The model under review builds one solid part; all positions refer to its coordinate system, in mm. Give positions to 0.01 mm unless a question says otherwise; leave off trailing zeros. Order: outer loops, then holes, each group sorted by start corner. A loop starts at its lowest first (then second) coordinate and runs counter-clockwise, first axis right, second up. Notation, with made-up numbers: (77, -2.75) - (117, -2.75) arc R24 ccw to (117, 28.25) - close; hole circle Ø3 at (-26, 31). An arc over 180 degrees is marked (long way). Use a Markdown table: item, result. Add a question column.
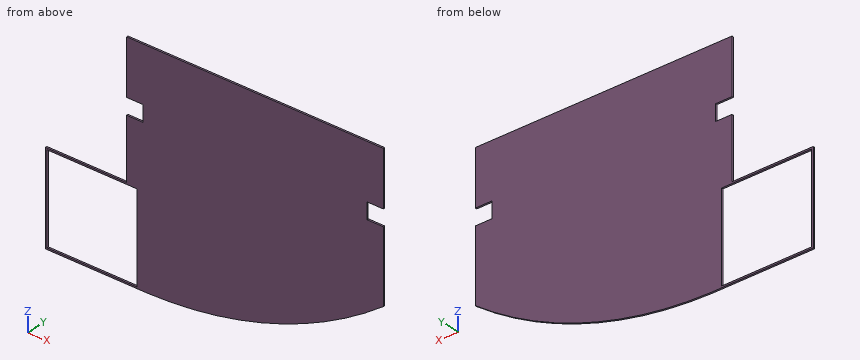
```python
from build123d import *

# Parameters (mm, degrees)
F0_W     = 139.7
F0_H     = 139.7
F1_DEPTH = 2.54
F2_W     = 25.4
F2_H     = 25.4
F3_DEPTH = 25.4
F4_W     = 25.4
F4_H     = 25.4
F5_DEPTH = 25.4


with BuildPart() as f1:
    # F0 (on Front) → F1 (new body)
    with BuildSketch(Plane.XZ):
        with BuildLine():
            Line((300.720289, 79.205069), (-98.059711, 79.205069))
            Line((-98.059711, 79.205069), (-98.059711, -128.566931))
            Line((-98.059711, -128.566931), (-224.297711, -128.566931))
            Line((-224.297711, -128.566931), (-224.297711, -273.346931))
            Line((-224.297711, -273.346931), (-82.057711, -273.346931))
            Line((-82.057711, -273.346931), (-64.778368, -273.346931))
            ThreePointArc((-64.778368, -273.346931), (128.230167, -239.372335), (300.720289, -146.346931))
            Line((300.720289, -146.346931), (300.720289, 79.205069))
        make_face()
        with Locations((-151.907711, -200.956931)):
            Rectangle(F0_W, F0_H, mode=Mode.SUBTRACT)
    extrude(amount=F1_DEPTH)

    # F2 (on face) → F3 (cut)
    with BuildSketch(Plane.XZ.offset(2.54)):
        with Locations((-85.359711, -19.854931)):
            Rectangle(F2_W, F2_H)
    extrude(amount=-F3_DEPTH, mode=Mode.SUBTRACT)

    # F4 (on face) → F5 (cut)
    with BuildSketch(Plane.XZ.offset(2.54)):
        with Locations((288.020289, -19.854931)):
            Rectangle(F4_W, F4_H)
    extrude(amount=-F5_DEPTH, mode=Mode.SUBTRACT)


solid = f1.part
```
Q1. Wall thickness on probe 1 along Z at (x, y) = (-137, -0.3); probe 2 along X at (y, z) = (-1.8, -197); probe 3 along X at (y, z) = (-1, -211.5): over which ranges is each line inside the solid? List them lowest first.
Q2. We need section C-C (x = 14.5). Write out the cut boundary in (y, z), plus the area to 3 significant figures.
Q3. Clearance check with flat-ended pins moving along their axes: P1, Ø0.8, axis at y = -1, z = -22.5, coming from the -X side; P2, Ø0.8, axis at x = -165, y = -0.5, coming from the +Z side; P3, Ø1.3, axis at y = -1.5, z = -101, coming from the -X side. State where each tip first meets the part, or that it passes through.
Q4. We need section B-B (y = -1.6). Write out the cut boundary in (x, z).
Q5. We need section D-D (x = 112.5). Write out the cut boundary in (y, z), plus the area to 3 significant figures.
Q6. We need section A-A (x = -106.5). Write out the cut boundary in (y, z), plus the area to 3 significant figures.
Here are the results:
| question | item | result |
|---|---|---|
| 1 | probe 1 | -273.35 to -270.81, -131.11 to -128.57 |
| 1 | probe 2 | -224.3 to -221.76, -82.06 to 223.31 |
| 1 | probe 3 | -224.3 to -221.76, -82.06 to 195.35 |
| 2 | outline | (-2.54, -267.08) - (0, -267.08) - (0, 79.21) - (-2.54, 79.21) - close |
| 2 | area | 880 mm2 |
| 3 | P1 | x = -72.66 |
| 3 | P2 | z = -128.57 |
| 3 | P3 | x = -98.06 |
| 4 | outline | (-224.3, -273.35) - (-64.78, -273.35) arc R614.37 ccw to (300.72, -146.35) - (300.72, -32.55) - (275.32, -32.55) - (275.32, -7.15) - (300.72, -7.15) - (300.72, 79.21) - (-98.06, 79.21) - (-98.06, -7.15) - (-72.66, -7.15) - (-72.66, -32.55) - (-98.06, -32.55) - (-98.06, -128.57) - (-224.3, -128.57) - close; hole (-221.76, -270.81) - (-82.06, -270.81) - (-82.06, -131.11) - (-221.76, -131.11) - close |
| 5 | outline | (-2.54, -244.6) - (0, -244.6) - (0, 79.21) - (-2.54, 79.21) - close |
| 5 | area | 822 mm2 |
| 6 | outline | (-2.54, -273.35) - (0, -273.35) - (0, -270.81) - (-2.54, -270.81) - close; (-2.54, -131.11) - (0, -131.11) - (0, -128.57) - (-2.54, -128.57) - close |
| 6 | area | 12.9 mm2 |
